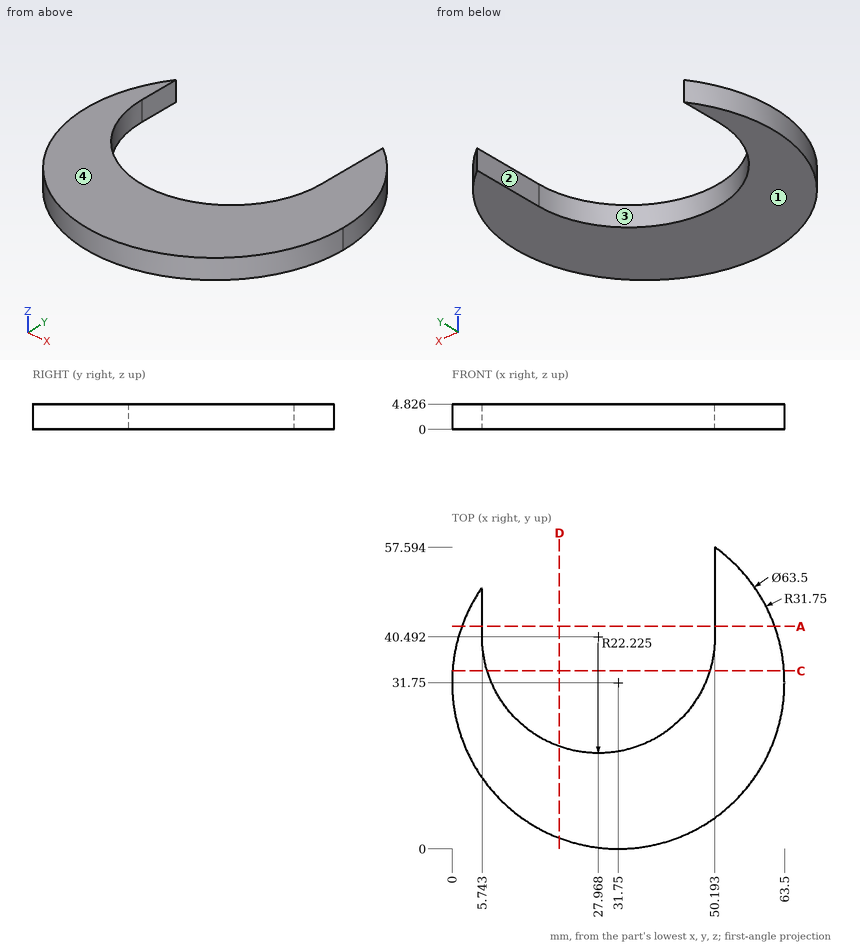
Here's the drawing with two shaded views (mm, measured from the low corner). I have some questions. A direction names the side the tool comes from. Round coordinates to 2 decimals unless told otherwise and drop trailing zeros. Order: outer loops, then holes, each group sorted by start corner. A loop starts at its lowest first (then second) coordinate and runs counter-clockwise, first axis right, second up. Notation, with made-up numbers: (12, 75) -> (33, 75) arc R10 cw to (33, 86) -> close; hole circle Ø10 at (-14, 87.25). An arc over 180 degrees is marked (long way). Use a Markdown table: item, result. Add a question column.
(1) For the marked faces 1 and 2, which set-ups out of +Z, -Z, +X, -X, +Y, -Y let a thin tool reach every point of the face, with its end or its side?
(2) I need wall thicknesses on line 1 along X through (y, z) = (46, 0.6); line 2 along X through (y, z) = (31, 1.45) (1 decimal); line 3 along Y through (x, z) = (30.5, 0.45) (1 decimal). Which ranges of each line are inside material? Lowest first, please.
(3) Suppose I cut it at C-C, the plane y = 34. Please give me the cut outline in (x, z).
(4) Suppose I cut it at D-D, the plane x = 20.5. Please give me the cut outline in (y, z).
(5) If we mould it in two halves opening along X, with no side actions, what happens to the marked faces 3 and 4? For each: released by +X, released by -X, zero draft, split by the parting line, or undercut.
(6) Suppose I cut it at A-A, the plane y = 42.5. Please give me the cut outline in (x, z) (1 decimal).
(7) For pin 1 Ø1.5 at (x, z) = (35.5, 2.5) entering from -Y; pin 2 Ø10 at (x, y) = (30, 16) entering from -Z, each with a flat end and sliding along its axis, tell me the tip position at first contact or that it passes through.
Verdict:
| question | item | result |
|---|---|---|
| 1 | face 1 | -Z, +X, -X, +Y, -Y |
| 1 | face 2 | +Z, -Z, +Y |
| 2 | line 1 | 3.38 to 5.74, 50.19 to 60.12 |
| 2 | line 2 | 0 to 7.9, 48.1 to 63.5 |
| 2 | line 3 | 0 to 18.4 |
| 3 | outline | (0.08, 0) -> (6.71, 0) -> (6.71, 4.83) -> (0.08, 4.83) -> close; (49.22, 0) -> (63.42, 0) -> (63.42, 4.83) -> (49.22, 4.83) -> close |
| 4 | outline | (2.06, 0) -> (19.56, 0) -> (19.56, 4.83) -> (2.06, 4.83) -> close |
| 5 | face 3 | undercut |
| 5 | face 4 | zero draft |
| 6 | outline | (1.9, 0) -> (5.7, 0) -> (5.7, 4.8) -> (1.9, 4.8) -> close; (50.2, 0) -> (61.6, 0) -> (61.6, 4.8) -> (50.2, 4.8) -> close |
| 7 | pin 1 | y = 0.14 |
| 7 | pin 2 | z = 0 |
